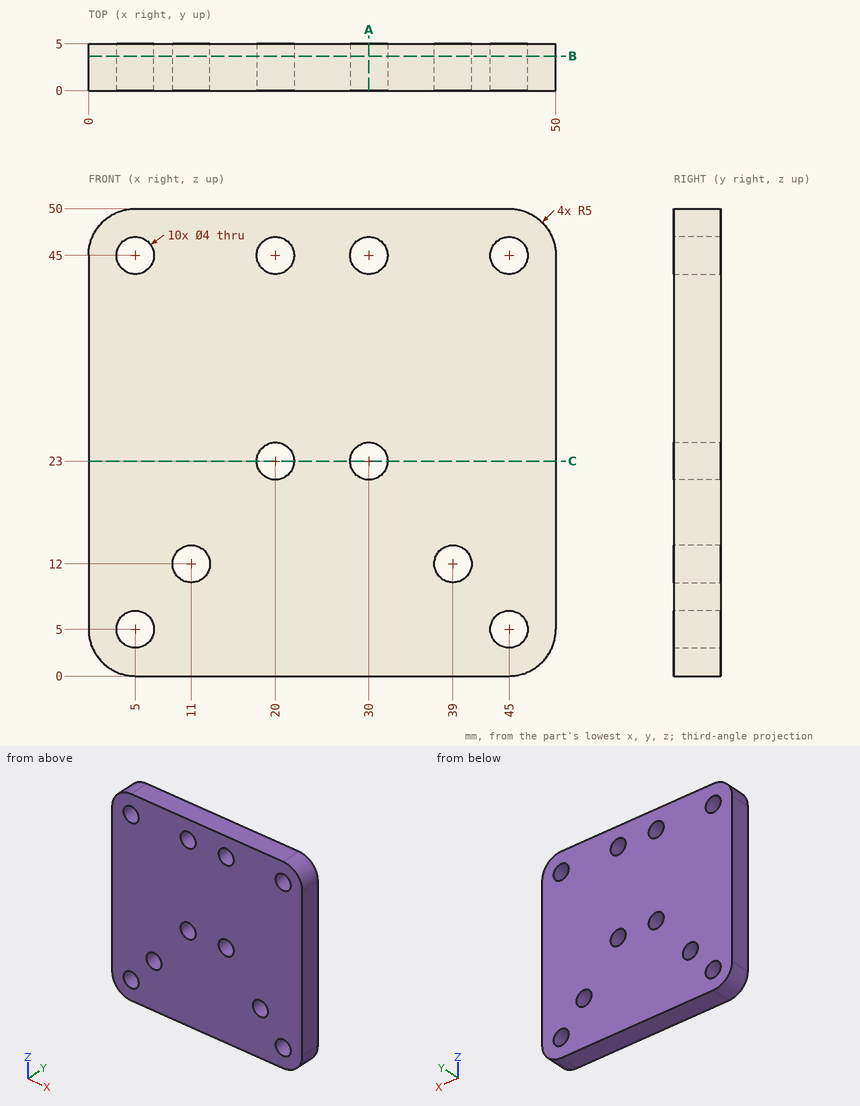
Design review of the part shown in the three views and the two pictorial views. Dimensions are in mm from the part's minimum x, y and z. Round coordinates to 2 decimals unless told otherwise and drop trailing zeros. Loops run counter-clockwise (first coordinate to the right, second up) from the corner with the lowest first, then second, coordinate; pieces in that order, holes last. Notation, with made-up numbers: M -39,35.25 L 4,35.25 A24 ccw 4,57.25 Z; hole C 17,-27.5 d1. An arc over 180 degrees is marked long. Write item = value, one per line.
Item 1: Insertion check: P1, Ø6.5, axis at x = 20, z = 23, coming from the -Y side; P2, Ø3, axis at x = 39, z = 12, coming from the -Y side. Each pin has a flat end and moves straight along its axis. Give the tip position at first contact, or say it passes through.
Return value:
P1 = 0
P2 = through
Item 2: For line 1 (X direction, y = 2.15, z = 45); line 2 (X direction, y = 1.95, z = 23); line 3 (X direction, y = 1.3, z = 12), list the stretches that pass through material, from the lowest coordinate up. Write a range as [from, to].
Return value:
line_1 = [0, 3], [7, 18], [22, 28], [32, 43], [47, 50]
line_2 = [0, 18], [22, 28], [32, 50]
line_3 = [0, 9], [13, 37], [41, 50]
Item 3: Take a section at C-C on z = 23. Write out the cut boundary in (x, y), then the cut area to 3 significant figures.
Return value:
outline = M 0,0 L 18,0 L 18,5 L 0,5 Z; M 22,0 L 28,0 L 28,5 L 22,5 Z; M 32,0 L 50,0 L 50,5 L 32,5 Z
area = 210 mm2
Item 4: Take a section at A-A on x = 30. Write out the cut boundary in (y, z).
Return value:
outline = M 0,0 L 5,0 L 5,21 L 0,21 Z; M 0,25 L 5,25 L 5,43 L 0,43 Z; M 0,47 L 5,47 L 5,50 L 0,50 Z
Item 5: Take a section at B-B on y = 3.7. State how many separate pieces and enclosed holes the cut face has, then the cut area to 3 significant figures.
Return value:
separate_pieces = 1
enclosed_holes = 10
area = 2,350 mm2
